```python
from build123d import *

# Parameters (mm, degrees)
BOSS_EXTRUDE10_DEPTH     = 0.5
BOSS_EXTRUDE10_DRAFT     = 45
BOSS_EXTRUDE11_DEPTH     = 11.499997616
SKETCH19_R               = 47.5
BOSS_EXTRUDE12_DEPTH     = 12.000000954
SKETCH20_R               = 19.75
BOSS_EXTRUDE13_DEPTH     = 1
SKETCH21_R               = 19.75
BOSS_EXTRUDE14_DEPTH     = 1
BOSS_EXTRUDE14_TAPER     = 45
SKETCH22_R               = 16
BOSS_EXTRUDE15_DEPTH     = 50
SKETCH28_R               = 57
BOSS_EXTRUDE17_DEPTH     = 0.5
BOSS_EXTRUDE17_DRAFT     = -45
BOSS_EXTRUDE18_DEPTH     = 205.500001907
F_9_0_9_DIAMETER_HOLE2_D = 9
CHAMFER5_SIZE            = 0.5
CHAMFER6_SIZE            = 0.25
SKETCH32_R               = 16
CUT_EXTRUDE1_DEPTH       = 311.604659233


with BuildPart() as part:
    # Sketch17 → Boss-Extrude10 (with draft: the straight prism first)
    with BuildSketch(Plane(origin=(0, 0, 15.249999762), x_dir=(-1, 0, 0), z_dir=(0, 0, -1))):
        with BuildLine():
            Line((-68.758451007, -77.559925727), (51.241548993, -77.559925727))
            ThreePointArc((51.241548993, -77.559925727), (56.433573045, -72.751949779), (61.241548993, -67.559925727))
            Line((61.241548993, -67.559925727), (61.241548993, 52.440074273))
            ThreePointArc((61.241548993, 52.440074273), (56.433573045, 57.632098325), (51.241548993, 62.440074273))
            Line((51.241548993, 62.440074273), (-68.758451007, 62.440074273))
            ThreePointArc((-68.758451007, 62.440074273), (-73.950475059, 57.632098325), (-78.758451007, 52.440074273))
            Line((-78.758451007, 52.440074273), (-78.758451007, -67.559925727))
            ThreePointArc((-78.758451007, -67.559925727), (-73.950475059, -72.751949779), (-68.758451007, -77.559925727))
        make_face()
    extrude(amount=-BOSS_EXTRUDE10_DEPTH)
    # Boss-Extrude10: the draft: its side faces are tilted about the plane it starts from
    boss_extrude10_sides = [part.faces().sort_by_distance(p)[0] for p in [
        (8.758451007, -77.559925727, 15.499999762),
        (-56.433573045, -72.751949779, 15.499999762),
        (-61.241548993, -7.559925727, 15.499999762),
        (-56.433573045, 57.632098325, 15.499999762),
        (8.758451007, 62.440074273, 15.499999762),
        (73.950475059, 57.632098325, 15.499999762),
        (78.758451007, -7.559925727, 15.499999762),
        (73.950475059, -72.751949779, 15.499999762),
    ]]
    draft(boss_extrude10_sides, Plane(origin=(0, 0, 15.249999762), x_dir=(-1, 0, 0), z_dir=(0, 0, -1)), BOSS_EXTRUDE10_DRAFT)

    # Sketch18 → Boss-Extrude11 (add)
    with BuildSketch(Plane.XY.offset(15.749999762)):
        with BuildLine():
            Line((-51.241548993, 62.440074273), (68.758451007, 62.440074273))
            ThreePointArc((68.758451007, 62.440074273), (73.950475059, 57.632098325), (78.758451007, 52.440074273))
            Line((78.758451007, 52.440074273), (78.758451007, -67.559925727))
            ThreePointArc((78.758451007, -67.559925727), (73.950475059, -72.751949779), (68.758451007, -77.559925727))
            Line((68.758451007, -77.559925727), (-51.241548993, -77.559925727))
            ThreePointArc((-51.241548993, -77.559925727), (-56.433573045, -72.751949779), (-61.241548993, -67.559925727))
            Line((-61.241548993, -67.559925727), (-61.241548993, 52.440074273))
            ThreePointArc((-61.241548993, 52.440074273), (-56.433573045, 57.632098325), (-51.241548993, 62.440074273))
        make_face()
    extrude(amount=BOSS_EXTRUDE11_DEPTH)

    # Sketch19 → Boss-Extrude12 (add)
    with BuildSketch(Plane.XY.offset(27.249997377)):
        with Locations((8.758451007, -7.559925727)):
            Circle(SKETCH19_R)
    extrude(amount=BOSS_EXTRUDE12_DEPTH)

    # Sketch20 → Boss-Extrude13 (add)
    with BuildSketch(Plane.XY.offset(39.249998331)):
        with Locations((8.758451007, -7.559925727)):
            Circle(SKETCH20_R)
    extrude(amount=BOSS_EXTRUDE13_DEPTH)

    # Sketch21 → Boss-Extrude14 (add)
    with BuildSketch(Plane.XY.offset(40.249998331)):
        with Locations((8.758451007, -7.559925727)):
            Circle(SKETCH21_R)
    extrude(amount=BOSS_EXTRUDE14_DEPTH, taper=BOSS_EXTRUDE14_TAPER)

    # Sketch22 → Boss-Extrude15 (add)
    with BuildSketch(Plane.XY.offset(41.249998331)):
        with Locations((8.758451007, -7.559925727)):
            Circle(SKETCH22_R)
    extrude(amount=BOSS_EXTRUDE15_DEPTH)


with BuildPart() as boss_extrude17_tool:
    # Sketch28 → Boss-Extrude17 (with draft: the straight prism first)
    with BuildSketch(Plane(origin=(0, 0, 15.249999762), x_dir=(-1, 0, 0), z_dir=(0, 0, -1))):
        with Locations((-8.758451007, -7.559925727)):
            Circle(SKETCH28_R)
    extrude(amount=BOSS_EXTRUDE17_DEPTH)
    # Boss-Extrude17: the draft: its side faces are tilted about the plane it starts from
    boss_extrude17_sides = [boss_extrude17_tool.faces().sort_by_distance(p)[0] for p in [
        (65.758451007, -7.559925727, 14.999999762),
    ]]
    draft(boss_extrude17_sides, Plane(origin=(0, 0, 15.249999762), x_dir=(-1, 0, 0), z_dir=(0, 0, -1)), BOSS_EXTRUDE17_DRAFT)


with BuildPart() as part_1:
    add(part.part)

    # Boss-Extrude17: add boss_extrude17_tool
    add(boss_extrude17_tool.part)

    # Sketch29 → Boss-Extrude18 (add)
    with BuildSketch(Plane(origin=(0, 0, 14.749999762), x_dir=(-1, 0, 0), z_dir=(0, 0, -1))):
        with BuildLine():
            Line((-44.813963761, -67.559925727), (27.297061748, -67.559925727))
            ThreePointArc((27.297061748, -67.559925727), (40.739023677, -57.05740041), (51.241548993, -43.615438482))
            Line((51.241548993, -43.615438482), (51.241548993, 28.495587027))
            ThreePointArc((51.241548993, 28.495587027), (40.739023677, 41.937548956), (27.297061748, 52.440074273))
            Line((27.297061748, 52.440074273), (-44.813963761, 52.440074273))
            ThreePointArc((-44.813963761, 52.440074273), (-58.25592569, 41.937548956), (-68.758451007, 28.495587027))
            Line((-68.758451007, 28.495587027), (-68.758451007, -43.615438482))
            ThreePointArc((-68.758451007, -43.615438482), (-58.25592569, -57.05740041), (-44.813963761, -67.559925727))
        make_face()
    extrude(amount=BOSS_EXTRUDE18_DEPTH)

    # Ø9.0 (9) Diameter Hole2 (through all)
    with Locations(Plane(origin=(0, 0, 15.249999762), x_dir=(-1, 0, 0), z_dir=(0, 0, -1))):
        with Locations((48.741548993, 49.940074273), (-66.258451007, 49.940074273), (-66.258451007, -65.059925727), (48.741548993, -65.059925727)):
            Hole(F_9_0_9_DIAMETER_HOLE2_D / 2)

    # Chamfer5
    chamfer5_edges = [part_1.edges().sort_by_distance(p)[0] for p in [
        (-53.241548993, 49.940074273, 15.249999762),
        (-56.433573045, 57.632098325, 27.249997377),
        (-61.241548993, -7.559925727, 27.249997377),
        (-56.433573045, -72.751949779, 27.249997377),
        (8.758451007, -77.559925727, 27.249997377),
        (73.950475059, -72.751949779, 27.249997377),
        (78.758451007, -7.559925727, 27.249997377),
        (73.950475059, 57.632098325, 27.249997377),
        (8.758451007, 62.440074273, 27.249997377),
        (-38.741548993, -7.559925727, 39.249998331),
        (58.25592569, 41.937548956, -190.750002146),
    ]]
    chamfer(chamfer5_edges, length=CHAMFER5_SIZE)

    # Chamfer6
    chamfer6_edges = [part_1.edges().sort_by_distance(p)[0] for p in [
        (-53.241548993, 49.940074273, 27.249997377),
    ]]
    chamfer(chamfer6_edges, length=CHAMFER6_SIZE)

    # Sketch32 → Cut-Extrude1 (cut, through all)
    with BuildSketch(Plane.XY.offset(99.249998331)):
        with Locations((8.758451007, -7.559925727)):
            Circle(SKETCH32_R)
    extrude(amount=-CUT_EXTRUDE1_DEPTH, mode=Mode.SUBTRACT)


solid = part_1.part
```
Design review of the part built by this model. Coordinates are the model's own, in mm. A direction names the side the tool comes from. Give positions to 0.01 mm unless a question says otherwise; leave off trailing zeros. Write each loop counter-clockwise with the first axis right and the second up, starting at its lowest first coordinate (ties: lowest second). Pieces come first, ordered by that corner, then holes. Notation, with made-up numbers: (-16, 66) - (-12, 66) arc R24 cw to (-12, 104) - close; hole circle Ø9 at (-5, -20). An arc over 180 degrees is marked (long way). Return JSON: item names as keys, results as strings. Group by question number.
(1) Machinability: for faces 1 (the flat face through (-51.242, -8, -87)), 2 (the flat face through (41, 40, 15.25)), 3 (the cylindrical face through (58.42, -56.89, -86.56)), 4 (the cylindrical face through (73.88, 57.7, 21.17)), 5 (the cylindrical face through (-56.363, -72.822, 21.173)), which of the approach directions +Z, -Z, +X, -X, +Y, -Y give a long, thin tool a straight path to every point of the face, cutting with its end or side? Answer none if there is none.
(2) Mouldability with a two-part tool opening along X and no side actions: class faces 6 (the conical face through (73.67, 57.49, 27.05)), 7 (the flat face through (-61.242, -8, 21)), 8 (the cylindrical face through (-49.717, 45.547, 21.454)) as +X half, -X half, draft (parallel to the pull), parting line (faces both ways), or undercut.
(3) Insertion check: pin 1 (5 mm diameter, centred on y = -9.5, z = -147, fed in from +X); pin 2 (2 mm diameter, centred on y = -7, z = -160, fed in from -X); pin 3 (1.5 mm diameter, centred on y = 45.5, z = -85, fed in from -X); pin 4 (7 mm diameter, centred on x = 66.26, y = 49.94, fed in from +Z). Each pin has a flat end and moves straight along its axis. Give the tip position at first contact, or say it passes through.
(4) We need section A-A, the plane z = -8. Give the boundary of the cut face in (x, y).
(5) To check wall thickness, follow probe 1 along Z at (x, y) = (60, 20.5); probe 2 along Y at (x, z) = (10, -49); probe 3 along Z at (x, y) = (-56, -40.5). State the ranges of each line that lie inside material, in increasing order.
(6) We need section B-B, the plane z = 20. Give the boundary of the cut face in (x, y).
Reported:
{
 "1": {"face 1": "-Z, -X, +Y, -Y", "face 2": "none", "face 3": "-Z, +X, -Y", "face 4": "+Z, +X, +Y", "face 5": "+Z, -X, -Y"},
 "2": {"face 6": "+X half", "face 7": "-X half", "face 8": "undercut"},
 "3": {"pin 1": "stops at x = 68.76", "pin 2": "stops at x = -51.24", "pin 3": "stops at x = -37.76", "pin 4": "passes through"},
 "4": {"outline": "(-51.24, -43.62) arc R70 ccw to (-27.3, -67.56) - (44.81, -67.56) arc R70 ccw to (68.76, -43.62) - (68.76, 28.5) arc R70 ccw to (44.81, 52.44) - (-27.3, 52.44) arc R70 ccw to (-51.24, 28.5) - close; hole circle Ø32 at (8.76, -7.56)"},
 "5": {"probe 1": "z = -190.75 to 14.75, 15.25 to 27.25", "probe 2": "y = -67.56 to -23.51, 8.39 to 52.44", "probe 3": "z = 15.25 to 27.25"},
 "6": {"outline": "(-61.24, -67.56) arc R92.2 ccw to (-51.24, -77.56) - (68.76, -77.56) arc R92.2 ccw to (78.76, -67.56) - (78.76, 52.44) arc R92.2 ccw to (68.76, 62.44) - (-51.24, 62.44) arc R92.2 ccw to (-61.24, 52.44) - close; hole circle Ø9 at (-48.74, -65.06); hole circle Ø9 at (-48.74, 49.94); hole circle Ø32 at (8.76, -7.56); hole circle Ø9 at (66.26, -65.06); hole circle Ø9 at (66.26, 49.94)"}
}
